Check sheet for the drawn part. Datum: minimum x, y, z corner. Units: mm. A direction names the side the tool comes from. Coordinates: 2 decimals unless noted, no trailing zeros. Write each loop counter-clockwise with the first axis right and the second up, starting at its lowest first coordinate (ties: lowest second). Pieces come first, ordered by that corner, then holes. Notation, with made-up numbers: (82, 53.25) -> (98, 53.25) arc R23 cw to (98, 80.25) -> close; hole circle Ø9 at (32, -19). An arc over 180 degrees is marked (long way). Answer in a Markdown table with one row per item. Add a question column.
1. Scan lines: L1, parallel to X at y = 26.5, z = 11.25; L2, parallel to X at y = 28.5, z = 7.5 (1 decimal); L3, parallel to Y at x = 9, z = 2. Record each from-to range of solid material in increasing order. Write a range as from..to.
2. Cross-section at C-C on x = 12.25. Record the cut outline in (y, z).
3. Depth check by flat-ended pin: P1, Ø5.5, axis at y = 29, z = 9.5, coming from the -X side; P2, Ø6, axis at y = 6.5, z = 10, coming from the -X side; P3, Ø4.5, axis at x = 11.5, z = 9.5, coming from the +Y side; P4, Ø2, axis at y = 18.5, z = 3, coming from the -X side (3 decimals). Enter the tip coordinate at first touch or a pass-through.
4. Cross-section at A-A on y = 27.5. Record the cut outline in (x, z) (1 decimal).
5. Set-up check for the marked faces 1, 2 and 3: record each of +Z, -Z, +X, -X, +Y, -Y from which the full face is reachable in a straight line by a thin tool's end or side.
6. Mould release check, pull along Z, two halves, no side actions. Record for the marked faces 4, 5 and 6: pulls with the +Z half, pulls with the -Z half, needs draft (parallel to the pull), parting line crosses it, or undercut.
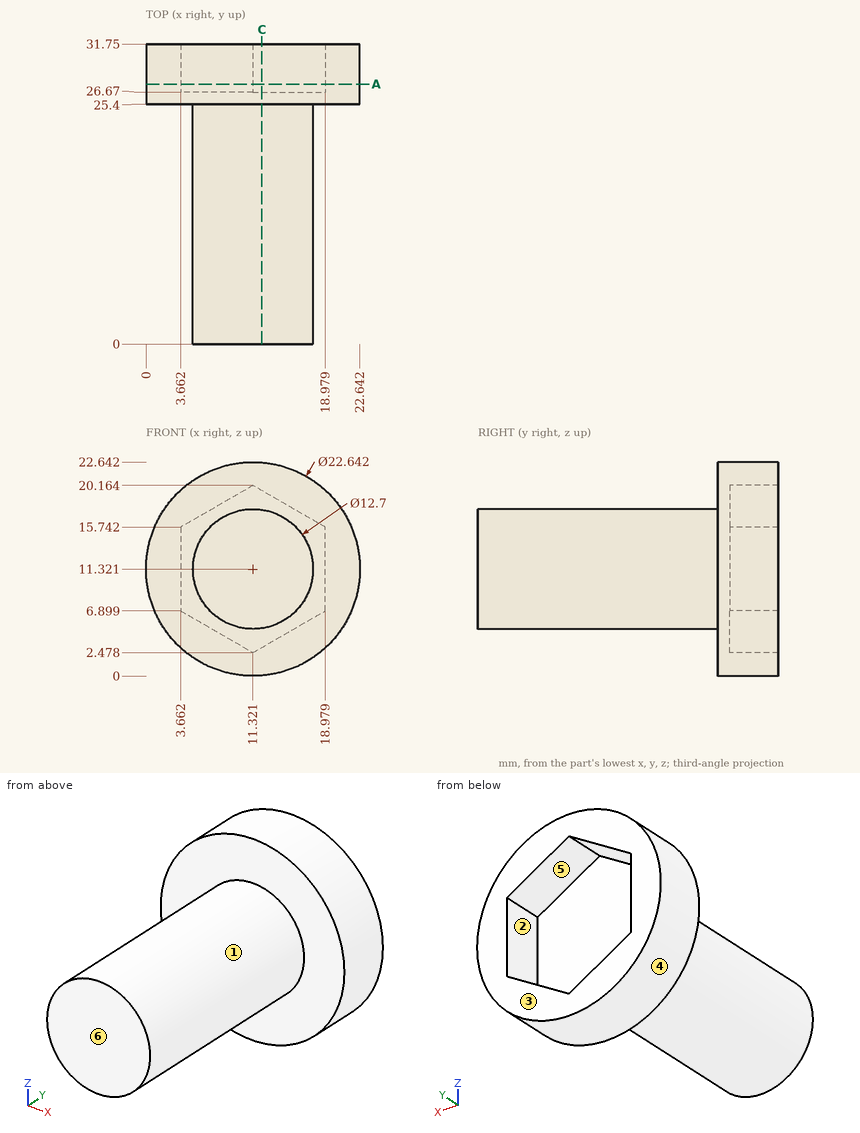
Results found:
| question | item | result |
|---|---|---|
| 1 | L1 | x = 0..22.64 |
| 1 | L2 | x = 0.7..3.7, 19..22 |
| 1 | L3 | y = 25.4..31.75 |
| 2 | outline | (0, 5.04) -> (25.4, 5.04) -> (25.4, 0.04) -> (31.75, 0.04) -> (31.75, 3.01) -> (26.67, 3.01) -> (26.67, 19.63) -> (31.75, 19.63) -> (31.75, 22.6) -> (25.4, 22.6) -> (25.4, 17.6) -> (0, 17.6) -> close |
| 3 | P1 | stops at x = 0 |
| 3 | P2 | stops at x = 4.97 |
| 3 | P3 | stops at y = 26.67 |
| 3 | P4 | passes through |
| 4 | outline | circle Ø22.6 at (11.3, 11.3); hole (3.7, 6.9) -> (11.3, 2.5) -> (19, 6.9) -> (19, 15.7) -> (11.3, 20.2) -> (3.7, 15.7) -> close |
| 5 | face 1 | -Y |
| 5 | face 2 | +Y |
| 5 | face 3 | +Z, -Z, +X, -X, +Y |
| 6 | face 4 | parting line crosses it |
| 6 | face 5 | undercut |
| 6 | face 6 | needs draft |
